```python
from build123d import *

# Parameters (mm, degrees)
F0_W          = 85
F0_H          = 180
F1_DEPTH      = 25
F2_R          = 15
F3_DEPTH      = 42.5
F3_DEPTH_BACK = 42.5
F4_W          = 55
F4_H          = 65
F5_DEPTH      = 180.001
F6_R          = 25
F7_DEPTH      = 10
F8_R          = 10
F9_DEPTH      = 15.001


with BuildPart() as f1:
    # F0 (on Top) → F1 (new body)
    with BuildSketch(Plane.XY):
        Rectangle(F0_W, F0_H)
    extrude(amount=F1_DEPTH)

    # F2 (on Right) → F3 (join, two sides)
    with BuildSketch(Plane.YZ) as f3_sk:
        with BuildLine():
            Line((0, 25), (-16.291713, 78.708287))
            ThreePointArc((-16.291713, 78.708287), (-45, 100), (-73.708287, 78.708287))
            Line((-73.708287, 78.708287), (-90, 25))
            Line((-90, 25), (0, 25))
        make_face()
        with Locations((-45, 70)):
            Circle(F2_R, mode=Mode.SUBTRACT)
    extrude(amount=F3_DEPTH)
    extrude(f3_sk.sketch, amount=-F3_DEPTH_BACK)

    # F4 (on face) → F5 (cut, through all)
    with BuildSketch(Plane.XZ.offset(90)):
        with Locations((0, 82.5)):
            Rectangle(F4_W, F4_H)
    extrude(amount=-F5_DEPTH, mode=Mode.SUBTRACT)

    # F6 (on face) → F7 (cut)
    with BuildSketch(Plane.XY.offset(25)):
        with Locations((0, 48)):
            Circle(F6_R)
    extrude(amount=-F7_DEPTH, mode=Mode.SUBTRACT)

    # F8 (on face) → F9 (cut, through all)
    with BuildSketch(Plane.XY.offset(15)):
        with Locations((0, 48)):
            Circle(F8_R)
    extrude(amount=-F9_DEPTH, mode=Mode.SUBTRACT)


solid = f1.part
```
CAD build for the part. Positions are in the model's coordinates, mm. A direction names the side the tool comes from. Give positions to 0.01 mm unless a question says otherwise; leave off trailing zeros. Order: outer loops, then holes, each group sorted by start corner. A loop starts at its lowest first (then second) coordinate and runs counter-clockwise, first axis right, second up.
(1) Saw through at A-A, the plane x = 0. Give the cut face in (y, z), then the cut area to 3 significant figures.
(2) Flat gauge pins, fed straight in: pin 1 (18 mm diameter, centred on y = -45, z = 70, fed in from +X); pin 2 (6 mm diameter, centred on x = -31.5, z = 27, fed in from -Y); pin 3 (5 mm diameter, centred on x = 29, y = 61.5, fed in from +Z). Where does each tip first touch, or does it go through?
(3) Saw through at C-C, the plane z = 18. Give the cut face in (x, y).
(4) Drill centre lines: L1, parallel to Y at x = 0, z = 18.5; L2, parallel to X at y = -63, z = 59; L3, parallel to Z at x = -14, y = -41. Where is each one in solid material? Low to high.
(5) Tool access for faces 1 (the flat face through (-27.5, -46, 86)), 2 (the cylindrical face through (35.105, -44.464, 99.995)), 3 (the cylindrical face through (-5.42, 23.594, 20.07)), 4 (the flat face through (-19, 66, 25)): list every direction of +Z, -Z, +X, -X, +Y, -Y with a clear straight run to the whole face (end or side of a thin tool).
(6) Saw through at D-D, the plane y = -45. Give the cut face in (x, z).
(7) Mould opens along Y. For faces 5 (the cylindrical face through (-34.895, -44.464, 99.995)), 6 (the flat face through (0, -46, 50)), 7 (the flat face through (11, 48, 15)) say: released by +Y, released by -Y, zero draft, split by the parting line, or undercut.
(8) Saw through at B-B, the plane y = 48. Give the cut face in (x, z), then the cut area to 4 significant figures.
Results found:
1. outline: (-90, 0) - (38, 0) - (38, 15) - (23, 15) - (23, 25) - (0, 25) - (-7.58, 50) - (-82.42, 50) - (-90, 25) - close; (58, 0) - (90, 0) - (90, 25) - (73, 25) - (73, 15) - (58, 15) - close
1. area: 5,760 mm2
2. pin 1: passes through
2. pin 2: stops at y = -90
2. pin 3: stops at z = 25
3. outline: (-42.5, -90) - (42.5, -90) - (42.5, 90) - (-42.5, 90) - close; hole circle Ø50 at (0, 48)
4. L1: y = -90 to 23, 73 to 90
4. L2: x = -42.5 to -27.5, 27.5 to 42.5
4. L3: z = 0 to 50
5. face 1: +Z, +Y, -Y
5. face 2: +Z, +X, -X
5. face 3: +Z
5. face 4: +Z, +X, -X, +Y
6. outline: (-42.5, 0) - (42.5, 0) - (42.5, 55) - (27.5, 55) - (27.5, 50) - (-27.5, 50) - (-27.5, 55) - (-42.5, 55) - close; (-42.5, 85) - (-27.5, 85) - (-27.5, 100) - (-42.5, 100) - close; (27.5, 85) - (42.5, 85) - (42.5, 100) - (27.5, 100) - close
7. face 5: split by the parting line
7. face 6: zero draft
7. face 7: undercut
8. outline: (-42.5, 0) - (-10, 0) - (-10, 15) - (-25, 15) - (-25, 25) - (-42.5, 25) - close; (10, 0) - (42.5, 0) - (42.5, 25) - (25, 25) - (25, 15) - (10, 15) - close
8. area: 1,325 mm2
